Can you work these out from the model? Positions are in its coordinate system, mm. A direction names the side the tool comes from. Give positions to 0.01 mm unless a question says otherwise; leave off trailing zeros. Loops run counter-clockwise (first coordinate to the right, second up) from the corner with the lowest first, then second, coordinate; pieces in that order, holes last.
from build123d import *

# Parameters (mm, degrees)
F1_DEPTH      = 25
F1_DEPTH_BACK = 25
F2_R          = 13
F3_R          = 4
F4_DEPTH      = 10
F5_R          = 2.5
F6_DEPTH      = 10
F7_R          = 2.5
F7_R_2        = 6.5
F8_DEPTH      = 10


with BuildPart() as f1:
    # F0 (on Front) → F1 (new body, two sides)
    with BuildSketch(Plane.XZ) as f1_sk:
        Polygon((-27.5, -35), (7.5, -35), (7.5, 35), (-37.5, 35), (-37.5, 30), (2.5, 30), (2.5, -30), (-27.5, -30), align=None)
    extrude(amount=F1_DEPTH)
    extrude(f1_sk.sketch, amount=-F1_DEPTH_BACK)

    # F2
    f2_edges = [f1.edges().sort_by_distance(p)[0] for p in [
        (7.5, 0, 35),
        (7.5, 0, -35),
        (2.5, 0, -30),
        (2.5, 0, 30),
    ]]
    fillet(f2_edges, radius=F2_R)

    # F3 (on face) → F4 (cut)
    with BuildSketch(Plane.XY.offset(35)):
        with Locations((-17.5, 0)):
            Circle(F3_R)
    extrude(amount=-F4_DEPTH, mode=Mode.SUBTRACT)

    # F5 (on face) → F6 (cut)
    with BuildSketch(Plane(origin=(0, 0, -35), x_dir=(1, 0, 0), z_dir=(0, 0, -1))):
        with Locations((-18, -14.5)):
            Circle(F5_R)
        with Locations((-18, 14.5)):
            Circle(F5_R)
    extrude(amount=-F6_DEPTH, mode=Mode.SUBTRACT)

    # F7 (on face) → F8 (cut)
    with BuildSketch(Plane.YZ.offset(7.5)):
        with Locations((11.5, -5.5)):
            Circle(F7_R)
        with Locations((-11.5, -5.5)):
            Circle(F7_R)
        with Locations((0, 3.5)):
            Circle(F7_R_2)
    extrude(amount=-F8_DEPTH, mode=Mode.SUBTRACT)


solid = f1.part
(1) Thinking about a two-plate mould opening in Z: for faces 5 (the cylindrical face through (3.591, -0.35, -31.293)), 6 (the cylindrical face through (-1.409, 0.35, -26.293)), 7 (the cylindrical face through (-20.5, 14.4, -32.5)), which applies, pulls with the +Z half, pulls with the -Z half, needs draft (parallel to the pull), parting line crosses it, or undercut?
Returned:
face 5: pulls with the -Z half
face 6: undercut
face 7: needs draft
(2) Suppose I cut it at D-D on y = 21.5. List the corners of the cut face in (x, z) for me, plus the area to 3 significant figures.
Returned:
outline: (-37.5, 30) - (-10.5, 30) arc R13 cw to (2.5, 17) - (2.5, -17) arc R13 cw to (-10.5, -30) - (-27.5, -30) - (-27.5, -35) - (-5.5, -35) arc R13 ccw to (7.5, -22) - (7.5, 22) arc R13 ccw to (-5.5, 35) - (-37.5, 35) - close
area: 700 mm2
(3) Suppose I cut it at B-B on y = 10. List the corners of the cut face in (x, z) for me.
Returned:
outline: (-37.5, 30) - (-10.5, 30) arc R13 cw to (2.5, 17) - (2.5, -3.5) - (7.5, -3.5) - (7.5, 22) arc R13 ccw to (-5.5, 35) - (-37.5, 35) - close; (-27.5, -35) - (-5.5, -35) arc R13 ccw to (7.5, -22) - (7.5, -7.5) - (2.5, -7.5) - (2.5, -17) arc R13 cw to (-10.5, -30) - (-27.5, -30) - close
(4) Suppose I cut it at C-C on x = -23.5. List the corners of the cut face in (y, z) for me.
Returned:
outline: (-25, -35) - (25, -35) - (25, -30) - (-25, -30) - close; (-25, 30) - (25, 30) - (25, 35) - (-25, 35) - close
(5) Will these pins go through, and if not, where does the flat tip stop? P1, Ø6, axis at y = -5, z = -7, coming from the -X side; P2, Ø1, axis at x = -30.5, y = -4, coming from the -Z side; P3, Ø8, axis at y = 0, z = 3.5, coming from the +X side; P4, Ø4, axis at y = -0.5, z = -32, coming from the -X side.
Returned:
P1: stops at x = 2.5
P2: stops at z = 30
P3: passes through
P4: stops at x = -27.5
(6) Which directions (+Z, -Z, +X, -X, +Y, -Y) give clear straight access to the entire face, cutting with the end or side of a thin tool? Please do faces 1 (the flat face through (2.5, 0, -4)), 2 (the flat face through (-25, 0, 35)), 3 (the flat face through (-27.5, 0, -32)), 4 (the cylindrical face through (-20.7, -2.4, 32.5)).
Returned:
face 1: -X, +Y, -Y
face 2: +Z, +X, -X, +Y, -Y
face 3: -Z, -X, +Y, -Y
face 4: +Z
(7) Please list where these lines run through material, in increasing order: probe 1 along Y at (x, z) = (-18, -33.85); probe 2 along Z at (x, y) = (-22.5, 9); probe 3 along Y at (x, z) = (5, 3).
Returned:
probe 1: y = -25 to -17, -12 to 12, 17 to 25
probe 2: z = -35 to -30, 30 to 35
probe 3: y = -25 to -6.48, 6.48 to 25
(8) Suppose I cut it at A-A on z = -7. List the corners of the cut face in (x, y) for me, plus the area to 3 significant figures.
Returned:
outline: (2.5, -25) - (7.5, -25) - (7.5, -13.5) - (2.5, -13.5) - close; (2.5, -9.5) - (7.5, -9.5) - (7.5, 9.5) - (2.5, 9.5) - close; (2.5, 13.5) - (7.5, 13.5) - (7.5, 25) - (2.5, 25) - close
area: 210 mm2
